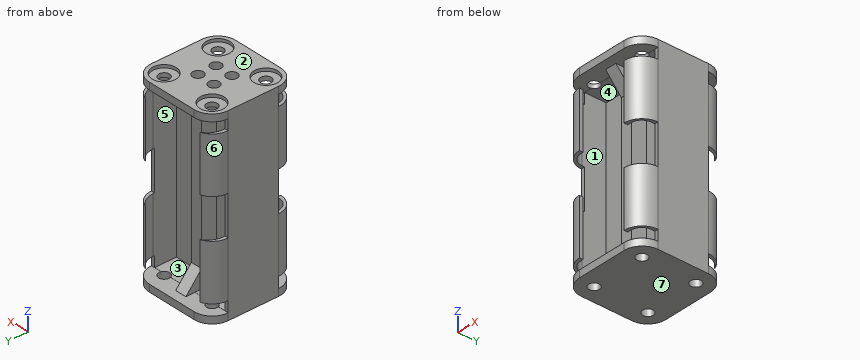
```python
from build123d import *

# Parameters (mm, degrees)
BOSS_EXTRU_1_DEPTH            = 62.4
ENL_V_MAT_EXTRU_1_DEPTH       = 27.6
ESQUISSE4_W                   = 3.6
ESQUISSE4_H                   = 10.193897514
ENL_V_MAT_EXTRU_2_DEPTH       = 62.4
ENL_V_MAT_EXTRU_5_REACH       = 74.618
ENL_V_START                   = -2.4
ESQUISSE7_R                   = 1.8
ENL_V_MAT_EXTRU_8_DEPTH       = 40
ESQUISSE8_R                   = 1.8
ENL_V_MAT_EXTRU_9_DEPTH       = 70
ENL_V_MAT_EXTRU_10_DEPTH      = 70
ENL_V_MAT_EXTRU_10_DEPTH_BACK = 70
ESQUISSE9_W                   = 3.6
ESQUISSE9_H                   = 8.374446498
ESQUISSE9_W_2                 = 13.276842972
ESQUISSE9_H_2                 = 11.709125621
ESQUISSE9_H_3                 = 11.001769443
ESQUISSE10_W                  = 28.8
ESQUISSE10_H                  = 2.4
BOSS_EXTRU_2_DEPTH            = 60
ESQUISSE12_W                  = 16.8
ESQUISSE12_H                  = 18.6
ENL_V_MAT_EXTRU_11_DEPTH      = 4
BOSS_EXTRU_3_DEPTH            = 1.92
BOSS_EXTRU_3_DEPTH_BACK       = 1.92
ESQUISSE14_R                  = 4
ENL_V_MAT_EXTRU_12_DEPTH      = 1


with BuildPart() as part:
    # Esquisse1 → Boss.-Extru.1 (new body)
    with BuildSketch(Plane.XY):
        with BuildLine():
            Line((8.4, 0), (-8.4, 0))
            ThreePointArc((-8.4, 0), (-12.642640687, -1.757359313), (-14.4, -6))
            Line((-14.4, -6), (-14.4, -22.8))
            ThreePointArc((-14.4, -22.8), (-12.642640687, -27.042640687), (-8.4, -28.8))
            Line((-8.4, -28.8), (8.4, -28.8))
            ThreePointArc((8.4, -28.8), (12.642640687, -27.042640687), (14.4, -22.8))
            Line((14.4, -22.8), (14.4, -6))
            ThreePointArc((14.4, -6), (12.642640687, -1.757359313), (8.4, 0))
        make_face()
    extrude(amount=-BOSS_EXTRU_1_DEPTH)

    # Esquisse2 → Enlèv. mat.-Extru.1 (cut)
    with BuildSketch(Plane(origin=(0, 0, 0), x_dir=(1, 0, 0), z_dir=(0, 1, 0))):
        Polygon((0, 2.4), (-8.4, 2.4), (-8.4, 60), (0, 60), (8.4, 60), (8.4, 2.4), align=None)
    extrude(amount=-ENL_V_MAT_EXTRU_1_DEPTH, mode=Mode.SUBTRACT)

    # Esquisse4 → Enlèv. mat.-Extru.2 (cut)
    with BuildSketch(Plane(origin=(14.4, 0, 0), x_dir=(0, 0, -1), z_dir=(1, 0, 0))):
        with Locations((4.161578514, -0.903051243)):
            Rectangle(ESQUISSE4_W, ESQUISSE4_H)
        Polygon((24.561578514, 4.193897514), (24.561578514, -6), (37.838421486, -6), (37.838421486, 4.193897514), (31.238421486, 4.193897514), (31.161578514, 4.193897514), align=None)
        with Locations((58.238421486, -0.903051243)):
            Rectangle(ESQUISSE4_W, ESQUISSE4_H)
    extrude(amount=-ENL_V_MAT_EXTRU_2_DEPTH, mode=Mode.SUBTRACT)

    # Enlèv. mat.-Extru.5: up to this face of the body (flat: up to its plane)
    enl_v_mat_extru_5_end = Plane(part.part.faces().sort_by_distance((0, -16.8, -60))[0])
    # Esquisse5 → Enlèv. mat.-Extru.5 (cut, up to the picked face)
    with BuildSketch(Plane.XY.offset(ENL_V_START), mode=Mode.PRIVATE) as enl_v_mat_extru_5_sk1:
        with BuildLine():
            Line((-7.2, 0.549733926), (7.2, 0.549733926))
            ThreePointArc((7.2, 0.549733926), (11.442640687, -1.207625387), (13.2, -5.450266074))
            Line((13.2, -5.450266074), (13.2, -13.850266074))
            Line((13.2, -13.850266074), (13.2, -14.949733926))
            Line((13.2, -14.949733926), (13.2, -23.349733926))
            Line((13.2, -23.349733926), (13.2, -24.06586829))
            ThreePointArc((13.2, -24.06586829), (12.164876788, -26.564876788), (9.66586829, -27.6))
            Line((9.66586829, -27.6), (0, -27.6))
            Line((0, -27.6), (-9.2, -27.6))
            ThreePointArc((-9.2, -27.6), (-12.028427125, -26.428427125), (-13.2, -23.6))
            Line((-13.2, -23.6), (-13.2, -23.349733926))
            Line((-13.2, -23.349733926), (-13.2, -14.949733926))
            Line((-13.2, -14.949733926), (-13.2, -13.850266074))
            Line((-13.2, -13.850266074), (-13.2, -5.450266074))
            ThreePointArc((-13.2, -5.450266074), (-11.442640687, -1.207625387), (-7.2, 0.549733926))
        make_face()
    enl_v_mat_extru_5_tool1 = split(extrude(enl_v_mat_extru_5_sk1.sketch, amount=-ENL_V_MAT_EXTRU_5_REACH, mode=Mode.PRIVATE), bisect_by=enl_v_mat_extru_5_end, keep=Keep.BOTH, mode=Mode.PRIVATE)
    add(enl_v_mat_extru_5_tool1.solids().sort_by(Axis((0.01246, -13.685747, -2.4), (0, 0, -1)))[0], mode=Mode.SUBTRACT)

    # Esquisse7 → Enlèv. mat.-Extru.8 (cut)
    with BuildSketch(Plane.XY):
        with Locations((3, -11.4)):
            Circle(ESQUISSE7_R)
        with Locations((-3, -11.4)):
            Circle(ESQUISSE7_R)
        with Locations((3, -17.4)):
            Circle(ESQUISSE7_R)
        with Locations((-3, -17.4)):
            Circle(ESQUISSE7_R)
    extrude(amount=-ENL_V_MAT_EXTRU_8_DEPTH, mode=Mode.SUBTRACT)

    # Esquisse8 → Enlèv. mat.-Extru.9 (cut)
    with BuildSketch(Plane.XY):
        with Locations((-9, -5.430075377)):
            Circle(ESQUISSE8_R)
        with Locations(Location((9, -5.430075377, 0), (0, 0, 341.541071197))):
            Circle(ESQUISSE8_R)
        with Locations((9, -23.369924623)):
            Circle(ESQUISSE8_R)
        with Locations((-9, -23.369924623)):
            Circle(ESQUISSE8_R)
    extrude(amount=-ENL_V_MAT_EXTRU_9_DEPTH, mode=Mode.SUBTRACT)

    # Esquisse9 → Enlèv. mat.-Extru.10 (cut, two sides: drawn at the far end of the back side and taken through both)
    with BuildSketch(Plane(origin=(0, 0, 0), x_dir=(0, 0, -1), z_dir=(1, 0, 0)).offset(-ENL_V_MAT_EXTRU_10_DEPTH_BACK)):
        with Locations((4.161578514, -26.987223249)):
            Rectangle(ESQUISSE9_W, ESQUISSE9_H)
        with Locations((31.2, -28.654562811)):
            Rectangle(ESQUISSE9_W_2, ESQUISSE9_H_2)
        with Locations((58.238421486, -28.300884722)):
            Rectangle(ESQUISSE9_W, ESQUISSE9_H_3)
    extrude(amount=ENL_V_MAT_EXTRU_10_DEPTH + ENL_V_MAT_EXTRU_10_DEPTH_BACK, mode=Mode.SUBTRACT)

    # Esquisse10 → Boss.-Extru.2 (add)
    with BuildSketch(Plane.XY):
        with Locations((0, -14.4)):
            Rectangle(ESQUISSE10_W, ESQUISSE10_H)
    extrude(amount=-BOSS_EXTRU_2_DEPTH)

    # Esquisse12 → Enlèv. mat.-Extru.11 (cut)
    with BuildSketch(Plane.XZ.offset(28.8)):
        with Locations((0, -47.138421486)):
            Rectangle(ESQUISSE12_W, ESQUISSE12_H)
        with Locations((0, -15.261578514)):
            Rectangle(ESQUISSE12_W, ESQUISSE12_H)
    extrude(amount=-ENL_V_MAT_EXTRU_11_DEPTH, mode=Mode.SUBTRACT)

    # Esquisse13 → Boss.-Extru.3 (add, two sides: drawn at the far end of the back side and taken through both)
    with BuildSketch(Plane(origin=(0, 0, 0), x_dir=(0, 0, -1), z_dir=(1, 0, 0)).offset(-BOSS_EXTRU_3_DEPTH_BACK)):
        Polygon((60.038421486, -3), (53.936448566, -8.235896166), (8.463551434, -8.235896166), (2.361578514, -3), (2.361578514, -25.8), (8.463551434, -20.564103834), (53.936448566, -20.564103834), (60.038421486, -25.8), align=None)
    extrude(amount=BOSS_EXTRU_3_DEPTH + BOSS_EXTRU_3_DEPTH_BACK)

    # Esquisse14 → Enlèv. mat.-Extru.12 (cut)
    with BuildSketch(Plane.XY):
        with Locations((-9, -5.430075377)):
            Circle(ESQUISSE14_R)
        with Locations(Location((9, -5.430075377, 0), (0, 0, 180))):
            Circle(ESQUISSE14_R)
        with Locations((9, -23.369924623)):
            Circle(ESQUISSE14_R)
        with Locations(Location((-9, -23.369924623, 0), (0, 0, 180))):
            Circle(ESQUISSE14_R)
    extrude(amount=-ENL_V_MAT_EXTRU_12_DEPTH, mode=Mode.SUBTRACT)


solid = part.part
```
For this review, take the finished solid that the model builds, in its own axes (mm). Face numbers are marked on the shaded views. A direction names the side the tool comes from. Give positions to 0.01 mm unless a question says otherwise; leave off trailing zeros. Write each loop counter-clockwise with the first axis right and the second up, starting at its lowest first coordinate (ties: lowest second). Pieces come first, ordered by that corner, then holes. Notation, with made-up numbers: M 58.5,-34.5 L 76.5,-34.5 A33 ccw 76.5,-3.5 Z; hole C -15,54 d4. An arc over 180 degrees is marked long. Answer as a JSON object with one key per item and string values. Group by question number.
Item 1: Consider section C-C on z = -58. Write out the cut boundary in (x, y), plus the area to 3 significant figures.
Item 2: Consider section B-B on y = -17.4. Write out the cut boundary in (x, z), plus the area to 3 significant figures.
Item 3: Consider section A-A on z = -11. Write out the cut boundary in (x, y).
Item 4: For probe 1 along Y at (x, z) = (3, -1.7); probe 2 along X at (y, z) = (-17.4, -1.6); probe 3 along X at (y, z) = (-9.5, -21), list the stretches that pass through material, from the lowest coordinate up. Write a range as [from, to].
Item 5: For pin 1 Ø1.3 at (y, z) = (-28, -11.5) entering from +X; pin 2 Ø8 at (x, z) = (1, -9) entering from +Y; pin 3 Ø1 at (x, z) = (-13.5, -31.5) entering from -Y, all flat-tipped, find the tip position at first contact; note any pin that passes through.
Item 6: Draft analysis for pull direction X (two halves, no side actions). For the marked faces 5, 6 and 7, state which applies: +X half, -X half, draft (parallel to the pull), parting line (faces both ways), or undercut.
Item 7: Tool access review of the marked faces 1, 2, 3 and 4: name each direction out of +Z, -Z, +X, -X, +Y, -Y from which nothing blocks a thin tool from reaching the whole face with its end or side.
Check result:
{
 "1": {"outline": "M -14.4,-22.8 L -13.2,-22.8 L -13.2,-15.6 L -1.92,-15.6 L -1.92,-24.05 L 1.92,-24.05 L 1.92,-15.6 L 13.2,-15.6 L 13.2,-22.8 L 14.4,-22.8 L 14.4,-6 L 13.2,-6 L 13.2,-13.2 L 1.92,-13.2 L 1.92,-4.75 L -1.92,-4.75 L -1.92,-13.2 L -13.2,-13.2 L -13.2,-6 L -14.4,-6 Z", "area": "169 mm^2"},
 "2": {"outline": "M -14.4,-62.4 L 14.4,-62.4 L 14.4,0 L 4.8,0 L 4.8,-2.4 L 13.2,-2.4 L 13.2,-60 L 1.92,-60 L 1.92,-2.36 L 1.2,-2.36 L 1.2,0 L -1.2,0 L -1.2,-2.36 L -1.92,-2.36 L -1.92,-60 L -13.2,-60 L -13.2,-2.4 L -4.8,-2.4 L -4.8,0 L -14.4,0 Z", "area": "480 mm^2"},
 "3": {"outline": "M -14.4,-22.8 A6 ccw -8.4,-28.8 L -8.4,-27.6 L -9.2,-27.6 A4 cw -13.2,-23.6 L -13.2,-15.6 L -1.92,-15.6 L -1.92,-20.56 L 1.92,-20.56 L 1.92,-15.6 L 13.2,-15.6 L 13.2,-24.07 A3.53 cw 9.67,-27.6 L 8.4,-27.6 L 8.4,-28.8 A6 ccw 14.4,-22.8 L 14.4,-6 A6 ccw 10.28,-0.3 A6 cw 13.2,-5.45 L 13.2,-13.2 L 1.92,-13.2 L 1.92,-8.24 L -1.92,-8.24 L -1.92,-13.2 L -13.2,-13.2 L -13.2,-5.45 A6 cw -10.28,-0.3 A6 ccw -14.4,-6 Z"},
 "4": {"probe 1": "y = [-28.8, -19.2], [-15.6, -13.2], [-9.6, 0]", "probe 2": "x = [-14.4, -4.8], [-1.2, 1.2], [4.8, 14.4]", "probe 3": "x = [-14.4, -13.2], [-1.92, 1.92], [13.2, 14.4]"},
 "5": {"pin 1": "stops at x = 12.31", "pin 2": "stops at y = -5.26", "pin 3": "stops at y = -22.8"},
 "6": {"face 5": "undercut", "face 6": "-X half", "face 7": "draft"},
 "7": {"face 1": "none", "face 2": "+Z, +X, -X, +Y, -Y", "face 3": "+Y", "face 4": "-Y"}
}
